```python
from build123d import *

# Parameters (mm, degrees)
HUB_NECK_SKETCH_R                   = 9
HUB_NECK_DEPTH                      = 10
RIM_CLAMP_FLANGE_SKETCH_R           = 18
RIM_CLAMP_FLANGE_DEPTH              = 3
AXLE_CLEARANCE_SKETCH_R             = 6.05
AXLE_CLEARANCE_DEPTH                = 10.2
RIM_BOLT_CLEARANCE_PATTERN_SKETCH_R = 1.7
RIM_BOLT_CLEARANCE_PATTERN_DEPTH    = 3.2
POSITIVE_HUB_PIN_BORE_SKETCH_R      = 1.5
POSITIVE_HUB_PIN_BORE_DEPTH         = 20


with BuildPart() as part:
    # Hub neck sketch → Hub neck (new body)
    with BuildSketch(Plane(origin=(0, -273, 0), x_dir=(1, 0, 0), z_dir=(0, 1, 0))):
        with Locations(Location((-19.009182883, 53.244882879, 0), (0, 0, 270))):
            Circle(HUB_NECK_SKETCH_R)
    extrude(amount=HUB_NECK_DEPTH)

    # Rim clamp flange sketch → Rim clamp flange (add)
    with BuildSketch(Plane(origin=(0, -266, 0), x_dir=(1, 0, 0), z_dir=(0, 1, 0))):
        with Locations(Location((-19.009182883, 53.244882879, 0), (0, 0, 270))):
            Circle(RIM_CLAMP_FLANGE_SKETCH_R)
    extrude(amount=RIM_CLAMP_FLANGE_DEPTH)

    # Axle clearance sketch → Axle clearance (cut)
    with BuildSketch(Plane(origin=(0, -273.1, 0), x_dir=(1, 0, 0), z_dir=(0, 1, 0))):
        with Locations(Location((-19.009182883, 53.244882879, 0), (0, 0, 270))):
            Circle(AXLE_CLEARANCE_SKETCH_R)
    extrude(amount=AXLE_CLEARANCE_DEPTH, mode=Mode.SUBTRACT)

    # Rim bolt clearance pattern sketch → Rim bolt clearance pattern (cut)
    with BuildSketch(Plane(origin=(0, -266.1, 0), x_dir=(1, 0, 0), z_dir=(0, 1, 0))):
        with Locations(Location((-7.009182883, 53.244882879, 0), (0, 0, 270))):
            Circle(RIM_BOLT_CLEARANCE_PATTERN_SKETCH_R)
        with Locations(Location((-25.009182883, 42.852578033, 0), (0, 0, 270))):
            Circle(RIM_BOLT_CLEARANCE_PATTERN_SKETCH_R)
        with Locations(Location((-25.009182883, 63.637187724, 0), (0, 0, 270))):
            Circle(RIM_BOLT_CLEARANCE_PATTERN_SKETCH_R)
    extrude(amount=RIM_BOLT_CLEARANCE_PATTERN_DEPTH, mode=Mode.SUBTRACT)

    # Positive hub pin bore sketch → Positive hub pin bore (cut)
    with BuildSketch(Plane(origin=(-45.972851797, 0, -26.542438361), x_dir=(0.5000000000000001, 0, -0.8660254037844386), z_dir=(0.8660254037844386, 0, 0.5000000000000001))):
        with Locations(Location((36.606829753, -269, 0), (0, 0, 180))):
            Circle(POSITIVE_HUB_PIN_BORE_SKETCH_R)
    extrude(amount=POSITIVE_HUB_PIN_BORE_DEPTH, mode=Mode.SUBTRACT)


solid = part.part
```
Work out the finished part from the listing and answer in its coordinate system (mm). Give positions to 0.01 mm unless a question says otherwise; leave off trailing zeros. Loops run counter-clockwise (first coordinate to the right, second up) from the corner with the lowest first, then second, coordinate; pieces in that order, holes last. Notation, with made-up numbers: (-39.75, 16.25) -> (-18.75, 16.25) arc R28 cw to (-18.75, 34.25) -> close; hole circle Ø4 at (-24, 38). An arc over 180 degrees is marked (long way). Use CSV: the item, a comma, the result in double quotes.
1. The mould has two halves that part along Z. Classify faces 1 (the cylindrical face through (-23.86, -264.521, -44.106)), 2 (the cylindrical face through (-23.86, -264.52, -64.89)), 3 (the flat face through (-14.8, -266, -61.5)), 4 (the cylindrical face through (-27.795, -269.549, -55.196)): +Z half, -Z half, draft (parallel to the pull), parting line (faces both ways), or undercut.
Found:
face 1,"undercut"
face 2,"undercut"
face 3,"draft"
face 4,"parting line"
2. The part is cut by section B-B (y = -265.5). Write down the section's boundary in (x, z), then the cut area to 3 significant figures.
Found:
outline,"circle Ø36 at (-19.01, -53.24); hole circle Ø3.4 at (-25.01, -63.64); hole circle Ø3.4 at (-25.01, -42.85); hole circle Ø12.1 at (-19.01, -53.24); hole circle Ø3.4 at (-7.01, -53.24)"
area,"876 mm^2"
3. The part is cut by section D-D (z = -50). State how many separate pieces and enclosed holes the cut face has, then the cut area to 3 significant figures.
Found:
separate pieces,"3"
enclosed holes,"0"
area,"113 mm^2"
4. Straight lines are drawn through the part: line 1 (Y direction, x = -11.5, z = -49); line 2 (Y direction, x = -17, z = -62.5); line 3 (X direction, y = -266.5, z = -55). For each, find the intervals that lie inside material, in ascending order.
Found:
line 1,"-273 to -270.5, -267.5 to -263"
line 2,"-266 to -263"
line 3,"-27.84 to -24.8, -13.22 to -10.18"
5. The part is cut by section C-C (z = -60). Write down the section's boundary in (x, y), then the cut area to 3 significant figures.
Found:
outline,"(-35.69, -266) -> (-24.96, -266) -> (-24.96, -273) -> (-13.06, -273) -> (-13.06, -266) -> (-2.32, -266) -> (-2.32, -263) -> (-35.69, -263) -> close"
area,"183 mm^2"
6. The part is cut by section A-A (x = -18.5). Write down the section's boundary in (y, z).
Found:
outline,"(-273, -62.23) -> (-266, -62.23) -> (-266, -71.24) -> (-263, -71.24) -> (-263, -59.27) -> (-273, -59.27) -> close; (-273, -47.22) -> (-263, -47.22) -> (-263, -35.25) -> (-266, -35.25) -> (-266, -44.26) -> (-273, -44.26) -> close"
7. Flat-ended cylindrical pins translate along their axes: pin 1 Ø1 at (y, z) = (-271.5, -50.5) entering from +X; pin 2 Ø4.5 at (x, z) = (-25.01, -63.64) entering from +Y; pin 3 Ø3 at (y, z) = (-270.5, -54.5) entering from -X; pin 4 Ø3 at (y, z) = (-266.5, -63) entering from +X. Find the tip coordinate at first contact, or state that the pin passes through.
Found:
pin 1,"x = -10.29"
pin 2,"y = -263"
pin 3,"x = -28.01"
pin 4,"x = -3.06"
